Geometry: see drawing. Coordinates: mm, zero at the bounding-box minimum. A direction names the side the tool comes from. Give positions to 0.01 mm unless a question says otherwise; leave off trailing zeros. Order: outer loops, then holes, each group sorted by start corner. A loop starts at its lowest first (then second) coordinate and runs counter-clockwise, first axis right, second up. Notation, with made-up numbers: (51, 69.25) - (67, 69.25) arc R21 cw to (67, 76.25) - close; hole circle Ø7 at (11.5, 81.5). An arc over 180 degrees is marked (long way). One line per item, written item: value.
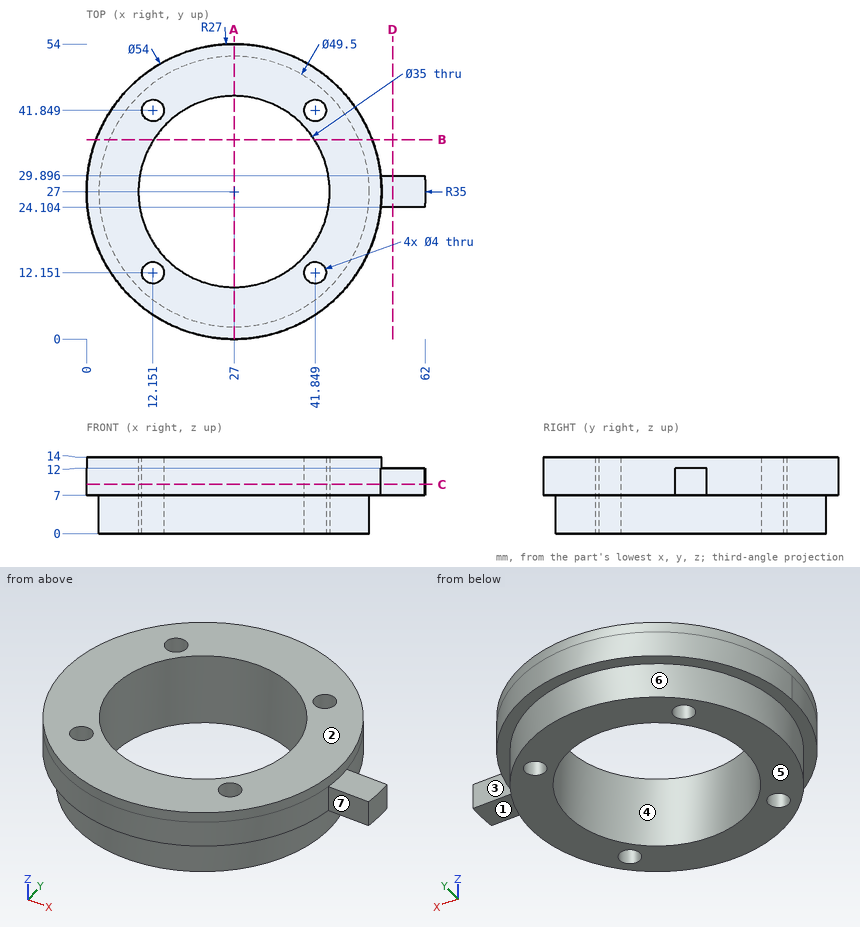
1) Set-up query: the marked faces 1, 2 and 3. Return all of +Z, -Z, +X, -X, +Y, -Y with unobstructed straight access to the full face (end or side cutting, diameter ignored); none if empty.
Answers below:
face 1: -Z
face 2: +Z, +X, -X, +Y, -Y
face 3: +Z, -Z, +X, +Y
2) Section A-A, the plane x = 27. Return loops of the section in (y, z).
Answers below:
outline: (0, 7) - (2.25, 7) - (2.25, 0) - (9.5, 0) - (9.5, 14) - (0, 14) - close; (44.5, 0) - (51.75, 0) - (51.75, 7) - (54, 7) - (54, 14) - (44.5, 14) - close
3) Mould query, pull axis Y, two halves, no side actions, for the marked faces 4, 5, 6 and 7. Classes: released by +Y, released by -Y, zero draft, split by the parting line, or undercut.
Answers below:
face 4: undercut
face 5: zero draft
face 6: split by the parting line
face 7: released by -Y
4) First-contact query: pin 1 (2.5 mm diameter, centred on x = 12.15, y = 12.15, fed in from +Z); pin 2 (8 mm diameter, centred on x = 17.5, z = 7.5, fed in from +Y); pin 3 (1.5 mm diameter, centred on x = 51.5, z = 10, fed in from +Y); pin 4 (1 mm diameter, centred on x = 35.5, z = 5.5, fed in from -Y). Flat tips, straight axial feed; report the tip coordinate or a pass-through.
Answers below:
pin 1: through
pin 2: y = 53.43
pin 3: y = 39.84
pin 4: y = 3.58
5) Material intervals for line 1 along Y through (x, z) = (13.5, 5.5) (1 decimal); line 2 along Y through (x, z) = (38, 2); line 3 along X through (y, z) = (17, 2), sorted ascending.
Answers below:
line 1: 6.3 to 10.7, 13.6 to 15.9, 38.1 to 40.4, 43.3 to 47.7
line 2: 4.83 to 13.39, 40.61 to 49.17
line 3: 4.36 to 12.64, 41.36 to 49.64
6) Section D-D, the plane x = 56. Return loops of the section in (y, z), then the cut area to 3 significant figures.
Answers below:
outline: (24.1, 7) - (29.9, 7) - (29.9, 12) - (24.1, 12) - close
area: 29.0 mm^2
7) Section C-C, the plane z = 9. Return loops of the section in (x, y), then the cut area to 3 significant figures.
Answers below:
outline: (53.84, 24.1) - (61.88, 24.1) arc R35 ccw to (61.88, 29.9) - (53.84, 29.9) arc R27 ccw (long way) to start; hole circle Ø35 at (27, 27); hole circle Ø4 at (12.15, 12.15); hole circle Ø4 at (12.15, 41.85); hole circle Ø4 at (41.85, 12.15); hole circle Ø4 at (41.85, 41.85)
area: 1,320 mm^2
8) Section B-B, the plane y = 36.5. Return loops of the section in (x, z).
Answers below:
outline: (1.73, 7) - (4.15, 7) - (4.15, 0) - (12.3, 0) - (12.3, 14) - (1.73, 14) - close; (41.7, 0) - (49.85, 0) - (49.85, 7) - (52.27, 7) - (52.27, 14) - (41.7, 14) - close
